from build123d import *

# Parameters (mm, degrees)
ESQUISSE1_R        = 67.8
BOSS_EXTRU_1_DEPTH = 20
ESQUISSE1_4_R      = 67.8
ESQUISSE1_4_R_2    = 50
BOSS_EXTRU_2_DEPTH = 10


with BuildPart() as part:
    # Esquisse1 → Boss.-Extru.1 (new body)
    with BuildSketch(Plane.XY):
        with BuildLine():
            Line((-188.729833462, 10), (-172.912878475, 10))
            ThreePointArc((-172.912878475, 10), (-125, 0), (-172.912878475, -10))
            Line((-172.912878475, -10), (-188.729833462, -10))
            ThreePointArc((-188.729833462, -10), (-167.842344673, -35.800149952), (-134.666666667, -36.944402673))
            ThreePointArc((-134.666666667, -36.944402673), (-91.362529225, -32.640861336), (-52.958333333, -53.107578843))
            ThreePointArc((-52.958333333, -53.107578843), (0, -75), (52.958333333, -53.107578843))
            ThreePointArc((52.958333333, -53.107578843), (91.362529225, -32.640861336), (134.666666667, -36.944402673))
            ThreePointArc((134.666666667, -36.944402673), (167.842344673, -35.800149952), (188.729833462, -10))
            Line((188.729833462, -10), (172.912878475, -10))
            ThreePointArc((172.912878475, -10), (125, 0), (172.912878475, 10))
            Line((172.912878475, 10), (188.729833462, 10))
            ThreePointArc((188.729833462, 10), (167.842344673, 35.800149952), (134.666666667, 36.944402673))
            ThreePointArc((134.666666667, 36.944402673), (91.362529225, 32.640861336), (52.958333333, 53.107578843))
            ThreePointArc((52.958333333, 53.107578843), (0, 75), (-52.958333333, 53.107578843))
            ThreePointArc((-52.958333333, 53.107578843), (-91.362529225, 32.640861336), (-134.666666667, 36.944402673))
            ThreePointArc((-134.666666667, 36.944402673), (-167.842344673, 35.800149952), (-188.729833462, 10))
        make_face()
        Circle(ESQUISSE1_R, mode=Mode.SUBTRACT)
    extrude(amount=BOSS_EXTRU_1_DEPTH)

    # Esquisse1_4 → Boss.-Extru.2 (add)
    with BuildSketch(Plane.XY):
        Circle(ESQUISSE1_4_R)
        Circle(ESQUISSE1_4_R_2, mode=Mode.SUBTRACT)
    extrude(amount=BOSS_EXTRU_2_DEPTH)


solid = part.part
Could you check a few things on this model? Use its own coordinates, in mm. A direction names the side the tool comes from. Round coordinates to 2 decimals unless told otherwise and drop trailing zeros. Order: outer loops, then holes, each group sorted by start corner. A loop starts at its lowest first (then second) coordinate and runs counter-clockwise, first axis right, second up. Notation, with made-up numbers: M 41,49.5 L 57,49.5 A16 cw 57,78.5 Z; hole C -35.5,58 d2. An arc over 180 degrees is marked long. One line per item, written item: value.
(1) Which directions (+Z, -Z, +X, -X, +Y, -Y) give clear straight access to the entire face, cutting with the end or side of a thin tool? Please do faces 1 (the flat face through (-45, -32, 0)), 2 (the flat face through (-5, -50, 10)), 3 (the cylindrical face through (168.27, 35.584, 9.86)), 4 (the flat face through (-181, 10, 10)), 5 (the flat face through (181, 10, 10)).
Ans:
face 1: -Z, +X, -X, +Y, -Y
face 2: +Z
face 3: +Z, -Z, +Y
face 4: +Z, -Z, -X
face 5: +Z, -Z, +X
(2) If we mould it in two halves opening along Y, with no side actions, what happens to faces 6 (the cylindrical face through (-49.971, 45.822, 14.93)), 7 (the cylindrical face through (-167.412, 36.011, 9.86)), 8 (the flat face through (-57, 39, 20)), 9 (the cylindrical face through (167.412, -36.011, 9.86))? For each: released by +Y, released by -Y, zero draft, split by the parting line, or undercut.
Ans:
face 6: undercut
face 7: released by +Y
face 8: zero draft
face 9: released by -Y
(3) Imagine slicing it at B-B (y = 0). Write out the boundary of the cut face in (x, z), and give its area (3 significant figures).
Ans:
outline: M -125,0 L -50,0 L -50,10 L -67.8,10 L -67.8,20 L -125,20 Z; M 50,0 L 125,0 L 125,20 L 67.8,20 L 67.8,10 L 50,10 Z
area: 2,640 mm^2
(4) I need wall thicknesses on line 1 along Y through (x, z) = (0, 4.25); line 2 along X through (y, z) = (-18.5, 15.25); line 3 along Y through (x, z) = (0, 14). Which ranges of each line are inside material? Lowest first, please. Write a range as from..to.
Ans:
line 1: y = -75..-50, 50..75
line 2: x = -185.46..-166.82, -133.18..-65.23, 65.23..133.18, 166.82..185.46
line 3: y = -75..-67.8, 67.8..75
(5) I'm going to push flat-ended pins straight in: P1, Ø2, axis at y = 31, z = 17.5, coming from the +X side; P2, Ø6, axis at y = 34.5, z = 3, coming from the +X side; P3, Ø4, axis at x = -19, z = 8.5, coming from the +Y side. Where does each tip first touch, or does it pass through?
Ans:
P1: stops at x = 176.46
P2: stops at x = 174.65
P3: stops at y = 73.05
(6) Imagine slicing it at C-C (z = 5). Write out the boundary of the cut face in (x, y), and give its area (3 significant figures).
Ans:
outline: M -188.73,-10 A40 ccw -134.67,-36.94 A75 cw -52.96,-53.11 A75 ccw 52.96,-53.11 A75 cw 134.67,-36.94 A40 ccw 188.73,-10 L 172.91,-10 A25 cw long 172.91,10 L 188.73,10 A40 ccw 134.67,36.94 A75 cw 52.96,53.11 A75 ccw -52.96,53.11 A75 cw -134.67,36.94 A40 ccw -188.73,10 L -172.91,10 A25 cw long -172.91,-10 Z; hole C 0,0 d100
area: 21,300 mm^2
(7) Imagine slicing it at A-A (x = -150). Write out the boundary of the cut face in (y, z).
Ans:
outline: M -40,0 L -25,0 L -25,20 L -40,20 Z; M 25,0 L 40,0 L 40,20 L 25,20 Z
(8) Imagine slicing it at D-D (y = 21). Write out the boundary of the cut face in (x, z), and give its area (3 significant figures).
Ans:
outline: M -184.04,0 L -163.56,0 L -163.56,20 L -184.04,20 Z; M -136.44,0 L -45.38,0 L -45.38,10 L -64.47,10 L -64.47,20 L -136.44,20 Z; M 45.38,0 L 136.44,0 L 136.44,20 L 64.47,20 L 64.47,10 L 45.38,10 Z; M 163.56,0 L 184.04,0 L 184.04,20 L 163.56,20 Z
area: 4,080 mm^2
